```python
from build123d import *

# Parameters (mm, degrees)
BOSS_EXTRUDE1_DEPTH = 6.35
SKETCH2_R           = 4.7625
BOSS_EXTRUDE2_DEPTH = 33.02
SKETCH3_OUTSIDE_W   = 65.944
SKETCH3_OUTSIDE_H   = 68.156
SKETCH3_OUTSIDE_R   = 7.1501
CUT_EXTRUDE1_DEPTH  = 20.32
CUT_EXTRUDE1_DRAFT  = -45
CHAMFER1_SIZE       = 0.254
CHAMFER1_SIZE2      = 0.022222121


with BuildPart() as part:
    # Sketch1 → Boss-Extrude1 (new body)
    with BuildSketch(Plane(origin=(0, 0, 0), x_dir=(1, 0, 0), z_dir=(0, 1, 0))):
        Polygon((0, 8.256224319), (-7.1501, 4.12811216), (-7.1501, -4.12811216), (0, -8.256224319), (7.1501, -4.12811216), (7.1501, 4.12811216), align=None)
    extrude(amount=BOSS_EXTRUDE1_DEPTH)

    # Sketch2 → Boss-Extrude2 (add)
    with BuildSketch(Plane.XZ):
        with Locations(Location((0, 0, 0), (0, 0, 90))):
            Circle(SKETCH2_R)
    extrude(amount=BOSS_EXTRUDE2_DEPTH)


with BuildPart() as cut_extrude1_tool:
    # Sketch3 outside → Cut-Extrude1 (with draft: the straight prism first)
    with BuildSketch(Plane(origin=(0, 6.35, 0), x_dir=(1, 0, 0), z_dir=(0, 1, 0))):
        Rectangle(SKETCH3_OUTSIDE_W, SKETCH3_OUTSIDE_H)
        Circle(SKETCH3_OUTSIDE_R, mode=Mode.SUBTRACT)
    extrude(amount=-CUT_EXTRUDE1_DEPTH)
    # Cut-Extrude1: the draft: its side faces are tilted about the plane it starts from
    cut_extrude1_sides = [cut_extrude1_tool.faces().sort_by_distance(p)[0] for p in [
        (0, -3.81, 34.078),
        (32.972, -3.81, 0),
        (0, -3.81, -34.078),
        (-32.972, -3.81, 0),
        (-7.1501, -3.81, 0),
    ]]
    draft(cut_extrude1_sides, Plane(origin=(0, 6.35, 0), x_dir=(1, 0, 0), z_dir=(0, 1, 0)), CUT_EXTRUDE1_DRAFT)


with BuildPart() as part_1:
    add(part.part)

    # Cut-Extrude1: cut by cut_extrude1_tool
    add(cut_extrude1_tool.part, mode=Mode.SUBTRACT)

    # Chamfer1
    chamfer1_edges = [part_1.edges().sort_by_distance(p)[0] for p in [
        (0, -33.02, -4.7625),
    ]]
    chamfer1_side = [part_1.faces().sort_by_distance(p)[0] for p in [
        (0, -16.51, -4.7625),
    ]]
    chamfer(chamfer1_edges, length=CHAMFER1_SIZE, length2=CHAMFER1_SIZE2, reference=chamfer1_side[0])


solid = part_1.part
```
Geometry check sheet. Reference: the model listing, model coordinates, mm. A direction names the side the tool comes from. Coordinates: 2 decimals unless noted, no trailing zeros. Write each loop counter-clockwise with the first axis right and the second up, starting at its lowest first coordinate (ties: lowest second). Pieces come first, ordered by that corner, then holes. Notation, with made-up numbers: M -5.5,-37.5 L 10.5,-37.5 A11 ccw 10.5,-29.5 Z; hole C 2,82.5 d10. An arc over 180 degrees is marked long. Use one line per item in the form item = value. Start each with the question number.
1) Section check A-A on y = -9. Enter the section's corners in (x, z) (1 decimal).
2) Set-up check for faces 1 (the cylindrical face through (2.9, -16.15, -3.78)), 2 (the conical face through (0, 6.1, -7.4)): record each of +Z, -Z, +X, -X, +Y, -Y from which the full face is reachable in a straight line by a thin tool's end or side.
3) Go/stop test with flat-tipped pins: pin 1 Ø1.5 at (x, y) = (4, -3) entering from +Z; pin 2 Ø3 at (x, y) = (5, -21) entering from +Z; pin 3 Ø3 at (y, z) = (-10, -1.5) entering from +X. Record where each tip stops, or that it passes through.
4) Thickness scan on probe 1 along Y at (x, z) = (4.25, 5.25); probe 2 along X at (y, z) = (-21, 0.5); probe 3 along Z at (x, y) = (-3.5, -18.5). Record the ranges inside material, lowest first. Write a range as from..to.
Responses:
q1.outline = C 0,0 d9.5
q2.face_1 = -Y
q2.face_2 = -Z, +Y
q3.pin_1 = 3.48
q3.pin_2 = 3.23
q3.pin_3 = 4.76
q4.probe_1 = 0..6.35
q4.probe_2 = -4.74..4.74
q4.probe_3 = -3.23..3.23
